```python
from build123d import *
from build123d.topology import SkipClean

# Parameters (mm, degrees)
SKETCH1_R           = 1.6
BOSS_EXTRUDE1_DEPTH = 6
BOSS_EXTRUDE3_START = 3
SKETCH7_R           = 1.6
BOSS_EXTRUDE3_DEPTH = 3
SKETCH8_R           = 1.6
BOSS_EXTRUDE4_DEPTH = 3
CHAMFER1_SIZE       = 2


with BuildPart() as part:
    # Sketch1 → Boss-Extrude1 (new body)
    with BuildSketch(Plane(origin=(0, 0, 0), x_dir=(1, 0, 0), z_dir=(0, 1, 0))):
        with BuildLine():
            Line((41.864892623, -74.106527494), (52.218230336, -84.960485214))
            ThreePointArc((52.218230336, -84.960485214), (62.095402371, -86.234826865), (65.834966495, -77.004543326))
            Line((65.834966495, -77.004543326), (61.8028085, -62.55664722))
            Line((61.8028085, -62.55664722), (67.581966942, -60.943784022))
            Line((67.581966942, -60.943784022), (74.892595581, -87.138988466))
            ThreePointArc((74.892595581, -87.138988466), (74.014994187, -93.014912457), (69.051034467, -96.279230281))
            ThreePointArc((69.051034467, -96.279230281), (57.637399431, -95.34940583), (47.97440772, -89.204307831))
            Line((47.97440772, -89.204307831), (37.523309535, -78.247862579))
            Line((37.523309535, -78.247862579), (41.864892623, -74.106527494))
        make_face()
        with Locations(Location((67.882250994, -89.09545443, 0), (0, 0, 270))):
            Circle(SKETCH1_R, mode=Mode.SUBTRACT)
    extrude(amount=BOSS_EXTRUDE1_DEPTH)

    # Sketch7 → Boss-Extrude3 (add)
    with SkipClean():  # the faces are left unmerged after this step: merging them gives an invalid solid
        with BuildSketch(Plane.XZ.offset(BOSS_EXTRUDE3_START)):
            with BuildLine():
                Line((37.523309535, 78.247862579), (41.864892623, 74.106527494))
                Line((41.864892623, 74.106527494), (61.8028085, 62.55664722))
                Line((61.8028085, 62.55664722), (67.581966942, 60.943784022))
                Line((67.581966942, 60.943784022), (74.892595581, 87.138988466))
                ThreePointArc((74.892595581, 87.138988466), (74.014994187, 93.014912457), (69.051034467, 96.279230281))
                ThreePointArc((69.051034467, 96.279230281), (57.637399431, 95.34940583), (47.97440772, 89.204307831))
                Line((47.97440772, 89.204307831), (37.523309535, 78.247862579))
            make_face()
            with Locations(Location((67.882250994, 89.09545443, 0), (0, 0, 270))):
                Circle(SKETCH7_R, mode=Mode.SUBTRACT)
            with Locations(Location((57.982756057, 79.195959493, 0), (0, 0, 270))):
                Circle(SKETCH7_R, mode=Mode.SUBTRACT)
        extrude(amount=-BOSS_EXTRUDE3_DEPTH)

    # Sketch8 → Boss-Extrude4 (add)
    with BuildSketch(Plane(origin=(0, 6, 0), x_dir=(1, 0, 0), z_dir=(0, 1, 0))):
        with BuildLine():
            Line((41.864892623, -74.106527494), (37.523309535, -78.247862579))
            Line((37.523309535, -78.247862579), (47.97440772, -89.204307831))
            ThreePointArc((47.97440772, -89.204307831), (57.637399431, -95.34940583), (69.051034467, -96.279230281))
            ThreePointArc((69.051034467, -96.279230281), (74.014994187, -93.014912457), (74.892595581, -87.138988466))
            Line((74.892595581, -87.138988466), (67.581966942, -60.943784022))
            Line((67.581966942, -60.943784022), (61.8028085, -62.55664722))
            Line((61.8028085, -62.55664722), (60.015359325, -63.592102685))
            Line((60.015359325, -63.592102685), (63.908580348, -77.542164392))
            ThreePointArc((63.908580348, -77.542164392), (61.023544246, -84.544233882), (53.530990497, -83.442395075))
            Line((53.530990497, -83.442395075), (43.643121603, -73.076413215))
            Line((43.643121603, -73.076413215), (41.864892623, -74.106527494))
        make_face()
        with Locations(Location((67.882250994, -89.09545443, 0), (0, 0, 90))):
            Circle(SKETCH8_R, mode=Mode.SUBTRACT)
    extrude(amount=BOSS_EXTRUDE4_DEPTH)

    # Chamfer1
    # the kernel refuses this chamfer: 2 mm, written as the material it takes off along each edge
    with BuildSketch(Plane(origin=(53.530990497, 6, 83.442395075), x_dir=(-0.7233236015009538, -0.02749587661058648, 0.689961552755735), z_dir=(-0.6902225142158023, 0, -0.7235971813582588))) as chamfer1_piece_1_section:
        Polygon((CHAMFER1_SIZE * 0.999621916911, CHAMFER1_SIZE * 0.0274958766106), (-CHAMFER1_SIZE * 0.0274958766106, CHAMFER1_SIZE * 0.999621916911), (0, 0), align=None)
    chamfer1_piece_1 = extrude(amount=19.468990959, mode=Mode.PRIVATE)
    chamfer1_piece_1 = split(chamfer1_piece_1, bisect_by=Plane(origin=(47.085687298, 6.664817027, 79.579765809), z_dir=(0.7235971813582587, 0, -0.6902225142158024)), keep=Keep.TOP, mode=Mode.PRIVATE)
    add(chamfer1_piece_1, mode=Mode.SUBTRACT)
    with BuildSketch(Plane(origin=(57.982756057, 6, 79.195959493), x_dir=(0.9631930737538318, 0, -0.26881053303887753), z_dir=(-0.26881053303887753, 0, -0.9631930737538318))) as chamfer1_piece_2_section:
        Polygon((6.152270455 + CHAMFER1_SIZE, 0), (6.152270455, -CHAMFER1_SIZE), (6.152270455, 0), align=None)
    chamfer1_piece_2 = revolve(axis=Axis((57.982756057, 6, 79.195959493), (0, -1, 0)), revolution_arc=151.945773521, mode=Mode.PRIVATE)
    chamfer1_piece_2 = split(chamfer1_piece_2, bisect_by=Plane(origin=(55.289387778, 6.562492794, 88.180143835), z_dir=(0.7235971813582587, 0, -0.6902225142158024)), keep=Keep.TOP, mode=Mode.PRIVATE)
    add(chamfer1_piece_2, mode=Mode.SUBTRACT)
    with BuildSketch(Plane(origin=(58.632768376, 6, 58.638048201), x_dir=(0.9628289067414894, -0.027495876610586514, -0.26870890032227024), z_dir=(0.2688105330388776, 0, 0.9631930737538319))) as chamfer1_piece_3:
        Polygon((CHAMFER1_SIZE * 0.999621916911, CHAMFER1_SIZE * 0.0274958766106), (-CHAMFER1_SIZE * 0.0274958766106, CHAMFER1_SIZE * 0.999621916911), (0, 0), align=None)
    extrude(amount=19.626507609, mode=Mode.SUBTRACT)


solid = part.part
```
Can you work these out from the model? Positions are in its coordinate system, mm. A direction names the side the tool comes from. Round coordinates to 2 decimals unless told otherwise and drop trailing zeros. Loops run counter-clockwise (first coordinate to the right, second up) from the corner with the lowest first, then second, coordinate; pieces in that order, holes last. Notation, with made-up numbers: (-32.75, 24.5) -> (23.25, 24.5) arc R28 ccw to (23.25, 58.5) -> close; hole circle Ø6 at (-2, -17). An arc over 180 degrees is marked (long way). Answer in a Markdown table with one row per item.
Item 1: Suppose I cut it at D-D, the plane y = -0.75. List the corners of the cut face in (x, z) for me.
Answer block:
| item | result |
|---|---|
| outline | (37.52, 78.25) -> (41.86, 74.11) -> (61.8, 62.56) -> (67.58, 60.94) -> (74.89, 87.14) arc R7.28 ccw to (69.05, 96.28) arc R23.84 ccw to (47.97, 89.2) -> close; hole circle Ø3.2 at (57.98, 79.2); hole circle Ø3.2 at (67.88, 89.1) |
Item 2: Suppose I cut it at C-C, the plane z = 76. List the corners of the cut face in (x, y) for me.
Answer block:
| item | result |
|---|---|
| outline | (39.88, -3) -> (71.78, -3) -> (71.78, 9) -> (63.48, 9) -> (63.48, 8) -> (65.55, 6) -> (65.55, 0) -> (43.67, 0) -> (43.67, 6) -> (46.43, 8) -> (46.43, 9) -> (39.88, 9) -> close |
Item 3: If I drill on probe 1 along X at (y, z) = (-2, 88); probe 2 along X at (y, z) = (7, 77.5); probe 3 along Y at (x, z) = (54, 67.5), over which ranges is the centre line in solid material (lowest first)?
Answer block:
| item | result |
|---|---|
| probe 1 | 46.83 to 66.72, 69.05 to 75.08 |
| probe 2 | 38.31 to 46.48, 64.93 to 72.2 |
| probe 3 | -3 to 0 |
Item 4: Will these pins go through, and if not, where does the flat tip stop? P1, Ø4, axis at y = 2.5, z = 84.5, coming from the -X side; P2, Ø6, axis at y = 4, z = 68.5, coming from the +X side; P3, Ø4, axis at x = 57.98, z = 79.2, coming from the -Y side; P4, Ø6, axis at x = 50.5, y = 7.5, coming from the +Z side.
Answer block:
| item | result |
|---|---|
| P1 | x = 41.58 |
| P2 | x = 70.53 |
| P3 | y = -3 |
| P4 | z = 93.51 |
Item 5: Suppose I cut it at A-A, the plane z = 88.5. List the corners of the cut face in (x, y) for me, plus the area to 3 significant figures.
Answer block:
| item | result |
|---|---|
| outline | (47.3, -3) -> (66.4, -3) -> (66.4, 9) -> (47.3, 9) -> close; (69.37, -3) -> (75.14, -3) -> (75.14, 9) -> (69.37, 9) -> close |
| area | 298 mm² |
Item 6: We'd pull the mould along Z, two halves only. Please class faces 4 (the flat face through (62.841, 6.986, 69.945)), 5 (the flat face through (42.676, 2.916, 83.649)), 6 (the flat face through (64.73, 2.92, 61.74)): released by +Z, released by -Z, zero draft, split by the parting line, or undercut.
Answer block:
| item | result |
|---|---|
| face 4 | undercut |
| face 5 | released by +Z |
| face 6 | released by -Z |
Item 7: On a 3-axis mill with a long thin cutter (end or side, diameter ignored), from which of +Z, -Z, +X, -X, +Y, -Y can I reach the whole of each face in a straight line? I mean faces 1 (the flat face through (47.759, 6.987, 78.859)), 2 (the flat face through (48.656, 8.493, 78.332)), 3 (the flat face through (57, 0, 75)). Say none if no direction works.
Answer block:
| item | result |
|---|---|
| face 1 | -Z |
| face 2 | -Z, +Y |
| face 3 | none |
Item 8: Suppose I cut it at B-B, the plane y = 5. List the corners of the cut face in (x, z) for me.
Answer block:
| item | result |
|---|---|
| outline | (37.52, 78.25) -> (41.86, 74.11) -> (52.22, 84.96) arc R8.15 cw to (65.83, 77) -> (61.8, 62.56) -> (67.58, 60.94) -> (74.89, 87.14) arc R7.28 ccw to (69.05, 96.28) arc R23.84 ccw to (47.97, 89.2) -> close; hole circle Ø3.2 at (67.88, 89.1) |
